Autodesk Inventor part; units mm, degrees
ref_plane "YZ Plane" through (0, 0, 0) normal (1, 0, 0) x (0, 1, 0)
ref_plane "XZ Plane" through (0, 0, 0) normal (0, 1, 0) x (-1, 0, 0)
ref_plane "XY Plane" through (0, 0, 0) normal (0, 0, 1) x (1, 0, 0)
sketch "Sketch1" plane through (0, 0, 0) normal (0, 0, 1) x (1, 0, 0)
  line L0 (-15.05, -12.5) -> (15.05, -12.5)
  line L1 (15.05, -12.5) -> (15.05, 12.5)
  line L2 (15.05, 12.5) -> (-15.05, 12.5)
  line L3 (-15.05, 12.5) -> (-15.05, -12.5)
  line L4 (-15.05, -12.5) -> (15.05, 12.5) construction
  line L5 (15.05, -12.5) -> (-15.05, 12.5) construction
  point P0 (0, 0)
  dimension "d0" = 30.1
  dimension "d1" = 25
extrude "Plate1" add sketch "Sketch1" along normal blind 1.5
sketch "Sketch6" plane through (0, 0, 1.5) normal (0, 0, 1) x (1, 0, 0)
  circle A0 centre (-8.15, 9.43) radius 0.7835
  circle A1 centre (-8.15, -6.57) radius 0.7835
  circle A2 centre (5.07, 8.43) radius 0.7835
  circle A3 centre (5.07, -5.57) radius 0.7835
  circle A4 centre (12.37, 1.43) radius 0.7835
  point P0 (0, 0)
hole "Hole2" at (-8.15, 9.43, 1.5) at (5.07, 8.43, 1.5) at (12.37, 1.43, 1.5) at (5.07, -5.57, 1.5) at (-8.15, -6.57, 1.5) direction (0, 0, -1) diameter 2.1 end through all
sketch "Sketch7" plane through (0, 0, 1.5) normal (0, 0, 1) x (1, 0, 0)
  circle A0 centre (-15.05, 1.43) radius 6.4
  circle A1 centre (-15.05, 1.43) radius 6.55
  point P0 (0, 0)
  dimension "d42" = 0.15
extrude "Cut1" cut sketch "Sketch7" against normal blind 1.5 contours A0 | A1
sketch "Sketch8" plane through (15.05, -11, 0) normal (0, -1, 0) x (1, 0, 0)
  line L0 (-30.1, 0) -> (0, 0)
  line L1 (0, 0) -> (0, 20)
  line L2 (0, 20) -> (-30.1, 20)
  line L3 (-30.1, 20) -> (-30.1, 0)
edge flange "Flange2" height 20 angle 90 thickness 1.5 bend radius 0.31 thickness toward (0, -1, 0) relief tear relief width 1.5 relief depth 0.75 edges at (0, -12.5, 1.5) wall of the first edge with corners at (-15.05, -11, 0) (15.05, -11, 0) (15.05, -11, 20) (-15.05, -11, 20)
bend "Bend2"
corner "Corner2"
sketch "Sketch9" plane through (-15.05, -11, 20) normal (0, 1, 0) x (1, 0, 0)
  circle A0 centre (10.05, 40.25) radius 40
  circle A1 centre (10.05, 40.25) radius 50
  point P0 (15.05, 20)
  dimension "d39" = 10
extrude "Cut2" cut sketch "Sketch9" against normal blind 1.5
fillet "Corner Round1" radius 1 2 edges at (15.05, 12.5, 0.75) (-15.05, 12.5, 0.75)
sketch "Sketch10" plane through (-15.05, -11, 1.81) normal (0, 1, 0) x (1, 0, 0)
  line L0 (30.1, 0) -> (0, 0)
  arc A0 (0, -16.6569) -> (30.1, -12.5521) centre (10.05, 22.06) ccw
  line L1 (15.05, 0) -> (15.05, -17.6263) construction
  point P0 (15.05, 1.81)
  point P1 (6.05, -5)
  point P2 (24.05, -5)
  point P3 (24.05, -12.5)
  point P4 (6.05, -14.5)
  dimension "d44" = 18
  dimension "d45" = 9.5
  dimension "d46" = 7.5
  dimension "d47" = 5
hole "Hole3" at (-9, -11, 6.81) at (9, -11, 6.81) at (9, -11, 14.31) at (-9, -11, 16.31) direction (0, -1, 0) diameter 2.1 end through all
equation "\"d27\" = Thickness"
equation "\"d40\" = Thickness"
equation "\"d2\" = Thickness"
equation "\"d29\" = BendReliefWidth"
equation "\"d30\" = BendReliefDepth"
equation "\"d31\" = MinimumRemnant"
equation "\"d32\" = TransitionRadius"
equation "\"d35\" = BendRadius"
equation "\"d36\" = CornerReliefSize"
equation "\"d37\" = GapSize"
equation "\"d38\" = JacobiRadiusSize"
equation "\"BendReliefWidth\" = Thickness"
equation "\"BendReliefDepth\" = 0.5 * Thickness"
equation "\"CornerReliefSize\" = 4 * Thickness"
equation "\"MinimumRemnant\" = 2 * Thickness"
equation "\"TransitionRadius\" = BendRadius"
equation "\"JacobiRadiusSize\" = BendRadius"
equation "\"GapSize\" = Thickness"
properties part number "axis_2_bottom_L_frame(top)" material "Aluminum 6061-AHC"
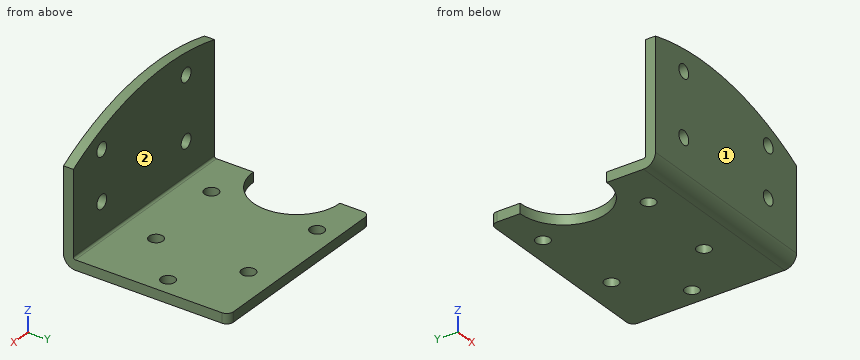
The model under review builds one solid part; all positions refer to its coordinate system, in mm. Face numbers are marked on the shaded views. A direction names the side the tool comes from. Give positions to 0.01 mm unless a question says otherwise; leave off trailing zeros. Order: outer loops, then holes, each group sorted by start corner. A loop starts at its lowest first (then second) coordinate and runs counter-clockwise, first axis right, second up. Notation, with made-up numbers: M 40,20.25 L 54,20.25 A36 ccw 54,55.25 Z; hole C 88,-18 d8. An arc over 180 degrees is marked long. Answer in a Markdown table with one row per item. Add a question column.
1. Add section C-C on y = 2. State the section outline as (x, z) points.
2. Add section B-B on x = 12.37. State the section outline as (y, z) points, plus the area to 3 significant figures.
3. Add section D-D on x = 9. State the section outline as (y, z) points.
4. To check wall thickness, follow line 1 along X through (y, z) = (-11.7, 6.81); line 2 along Z through (x, y) = (-9, -11.9); line 3 along Y through (x, z) = (-3, 9). State the ranges of each line that lie inside material, in increasing order.
5. Machinability: for the marked faces 1 and 2, which of the approach directions +Z, -Z, +X, -X, +Y, -Y give a long, thin tool a straight path to every point of the face, cutting with its end or side? Answer none if there is none.
6. For pin 1 Ø2 at (x, z) = (-3.5, 14) entering from +Y; pin 2 Ø8 at (x, y) = (-10.5, -6.5) entering from +Z; pin 3 Ø1.9 at (x, z) = (9, 14.31) entering from -Y; pin 4 Ø2.5 at (x, z) = (9, 6.81) entering from -Y, all flat-tipped, find the tip position at first contact; note any pin that passes through.
7. Add section A-A on z = 15.75. State the section outline as (x, y) points, plus the area to 3 significant figures.
The answers:
| question | item | result |
|---|---|---|
| 1 | outline | M -8.52,0 L 11.49,0 L 11.49,1.5 L -8.52,1.5 Z; M 13.25,0 L 15.05,0 L 15.05,1.5 L 13.25,1.5 Z |
| 2 | outline | M -12.5,1.81 A1.81 ccw -10.69,0 L 0.38,0 L 0.38,1.5 L -10.69,1.5 A0.31 cw -11,1.81 L -11,15.78 L -12.5,15.78 Z; M 2.48,0 L 12.5,0 L 12.5,1.5 L 2.48,1.5 Z |
| 2 | area | 55.1 mm2 |
| 3 | outline | M -12.5,1.81 A1.81 ccw -10.69,0 L 12.5,0 L 12.5,1.5 L -10.69,1.5 A0.31 cw -11,1.81 L -11,5.76 L -12.5,5.76 Z; M -12.5,7.86 L -11,7.86 L -11,13.26 L -12.5,13.26 Z; M -12.5,15.36 L -11,15.36 L -11,17.22 L -12.5,17.22 Z |
| 4 | line 1 | -15.05 to -10.05, -7.95 to 7.95, 10.05 to 15.05 |
| 4 | line 2 | 0.46 to 5.76, 7.86 to 15.26, 17.36 to 19.55 |
| 4 | line 3 | -12.5 to -11 |
| 5 | face 1 | +Z, -Z, +X, -X, -Y |
| 5 | face 2 | +Z, +X, -X, +Y |
| 6 | pin 1 | y = -11 |
| 6 | pin 2 | z = 1.5 |
| 6 | pin 3 | through |
| 6 | pin 4 | y = -12.5 |
| 7 | outline | M -15.05,-12.5 L -9.89,-12.5 L -9.89,-11 L -15.05,-11 Z; M -8.11,-12.5 L 12.44,-12.5 L 12.44,-11 L -8.11,-11 Z |
| 7 | area | 38.6 mm2 |
